```python
from build123d import *

# Parameters (mm, degrees)
CROQUIS1_W              = 68
CROQUIS1_H              = 64
CROQUIS1_W_2            = 61.625
CROQUIS1_H_2            = 58
SALIENTE_EXTRUIR1_DEPTH = 25
SALIENTE_EXTRUIR2_DEPTH = 160
SALIENTE_EXTRUIR3_DEPTH = 61
SALIENTE_EXTRUIR5_DEPTH = 3
CROQUIS4_W              = 100
CROQUIS4_H              = 30
CORTAR_EXTRUIR1_DEPTH   = 83
CHAFL_N1_SIZE           = 2
CHAFL_N1_SIZE2          = 57.272506566
CROQUIS1_2_W            = 68
CROQUIS1_2_H            = 64
CROQUIS1_2_W_2          = 61.625
CROQUIS1_2_H_2          = 58
SALIENTE_EXTRUIR6_DEPTH = 5
CROQUIS5_W              = 40
CROQUIS5_H              = 60
CORTAR_EXTRUIR2_DEPTH   = 90
CROQUIS1_4_W            = 68
CROQUIS1_4_H            = 10
CROQUIS1_4_R            = 2
SALIENTE_EXTRUIR7_DEPTH = 5
CROQUIS6_W              = 75.447981844
CROQUIS6_H              = 15
CORTAR_EXTRUIR3_DEPTH   = 5
CHAFL_N2_SIZE           = 30
CHAFL_N2_SIZE_2         = 1.572233378
CHAFL_N3_SIZE           = 5
CHAFL_N3_SIZE2          = 0.881634904
CROQUIS7_W              = 58
CROQUIS7_H              = 20
CORTAR_EXTRUIR4_DEPTH   = 40
CROQUIS8_W              = 58
CROQUIS8_H              = 40
CORTAR_EXTRUIR5_DEPTH   = 10
REDONDEO2_R             = 5
CORTAR_EXTRUIR6_DEPTH   = 70
REDONDEO5_R             = 5


with BuildPart() as part:
    # Croquis1 → Saliente-Extruir1 (new body)
    with BuildSketch(Plane(origin=(0, 0, 0), x_dir=(1, 0, 0), z_dir=(0, 1, 0))):
        Rectangle(CROQUIS1_W, CROQUIS1_H)
        Rectangle(CROQUIS1_W_2, CROQUIS1_H_2, mode=Mode.SUBTRACT)
    extrude(amount=SALIENTE_EXTRUIR1_DEPTH)

    # Croquis2 → Saliente-Extruir2 (add)
    with BuildSketch(Plane(origin=(0, 25, 0), x_dir=(1, 0, 0), z_dir=(0, 1, 0))):
        Polygon((0, 29), (0, 32), (34, 32), (34, -32), (0, -32), (0, -29), (30.8125, -29), (30.8125, 29), align=None)
    extrude(amount=SALIENTE_EXTRUIR2_DEPTH)



with BuildPart() as body_2:
    # Croquis3 → Saliente-Extruir3 (new body)
    with BuildSketch(Plane(origin=(0, 0, 29), x_dir=(-1, 0, 0), z_dir=(0, 0, -1))):
        Polygon((0, 155), (5, 155), (2, 85), (0, 85), align=None)
    extrude(amount=SALIENTE_EXTRUIR3_DEPTH)


with BuildPart() as part_1:
    add(part.part)

    add(body_2.part)  # Saliente-Extruir5 merges body 2
    # Croquis3<4> → Saliente-Extruir5 (add)
    with BuildSketch(Plane(origin=(0, 0, 29), x_dir=(-1, 0, 0), z_dir=(0, 0, -1))):
        Polygon((0, 155), (5, 155), (2, 85), (0, 85), align=None)
    extrude(amount=-SALIENTE_EXTRUIR5_DEPTH)

    # Croquis4 → Cortar-Extruir1 (cut)
    with BuildSketch(Plane(origin=(0, 0, -32), x_dir=(-1, 0, 0), z_dir=(0, 0, -1))):
        with Locations((19, 170)):
            Rectangle(CROQUIS4_W, CROQUIS4_H)
    extrude(amount=-CORTAR_EXTRUIR1_DEPTH, mode=Mode.SUBTRACT)

    # Chaflán1
    chafl_n1_edges = [part_1.edges().sort_by_distance(p)[0] for p in [
        (0, 155, 0),
    ]]
    chafl_n1_side = [part_1.faces().sort_by_distance(p)[0] for p in [
        (13, 155, -31.26569761),
    ]]
    chamfer(chafl_n1_edges, length=CHAFL_N1_SIZE, length2=CHAFL_N1_SIZE2, reference=chafl_n1_side[0])

    # Croquis1<2> → Saliente-Extruir6 (add)
    # profile 1 of 2: a face of its own
    with BuildSketch(Plane(origin=(0, 0, 0), x_dir=(1, 0, 0), z_dir=(0, 1, 0))):
        Rectangle(CROQUIS1_2_W, CROQUIS1_2_H)
        Rectangle(CROQUIS1_2_W_2, CROQUIS1_2_H_2, mode=Mode.SUBTRACT)
    # profile 2 of 2: a face of its own
    with BuildSketch(Plane(origin=(0, 0, 0), x_dir=(1, 0, 0), z_dir=(0, 1, 0))):
        Rectangle(CROQUIS1_2_W_2, CROQUIS1_2_H_2)
    extrude(amount=SALIENTE_EXTRUIR6_DEPTH)

    # Croquis5 → Cortar-Extruir2 (cut)
    with BuildSketch(Plane(origin=(0, 0, -32), x_dir=(-1, 0, 0), z_dir=(0, 0, -1))):
        with Locations((-11, 55)):
            Rectangle(CROQUIS5_W, CROQUIS5_H)
    extrude(amount=-CORTAR_EXTRUIR2_DEPTH, mode=Mode.SUBTRACT)

    # Croquis1<4> → Saliente-Extruir7 (add)
    # profile 1 of 2: a face of its own
    with BuildSketch(Plane(origin=(0, 0, 0), x_dir=(1, 0, 0), z_dir=(0, 1, 0))):
        with Locations((0, 37)):
            Rectangle(CROQUIS1_4_W, CROQUIS1_4_H)
        with Locations(Location((0, 37, 0), (0, 0, 270))):
            Circle(CROQUIS1_4_R, mode=Mode.SUBTRACT)
    # profile 2 of 2: a face of its own
    with BuildSketch(Plane(origin=(0, 0, 0), x_dir=(1, 0, 0), z_dir=(0, 1, 0))):
        with Locations((0, -37)):
            Rectangle(CROQUIS1_4_W, CROQUIS1_4_H)
        with Locations(Location((0, -37, 0), (0, 0, 270))):
            Circle(CROQUIS1_4_R, mode=Mode.SUBTRACT)
    extrude(amount=SALIENTE_EXTRUIR7_DEPTH)

    # Croquis6 → Cortar-Extruir3 (cut)
    with BuildSketch(Plane.ZY.offset(-31)):
        with Locations((5.723990922, 177.5)):
            Rectangle(CROQUIS6_W, CROQUIS6_H)
    extrude(amount=-CORTAR_EXTRUIR3_DEPTH, mode=Mode.SUBTRACT)

    # Chaflán2
    # the kernel refuses this chamfer: 30, 1.572233378 mm, written as the material it takes off along each edge
    with BuildSketch(Plane(origin=(31, 170, -109.996046635), x_dir=(-0.002013023422382327, -0.9999979738662979, 0), z_dir=(0, 0, 1))) as chafl_n2_piece_1_section:
        Polygon((CHAFL_N2_SIZE * 0.999997973866, CHAFL_N2_SIZE * 0.00201302342238), (-CHAFL_N2_SIZE_2 * 0.00201302342301, CHAFL_N2_SIZE_2 * 0.999997974179), (0, 0), align=None)
    chafl_n2_piece_1 = extrude(amount=219.992093269, mode=Mode.PRIVATE)
    chafl_n2_piece_1 = split(chafl_n2_piece_1, bisect_by=Plane(origin=(31.611424092, 155, 0), z_dir=(0, 1, 0)), keep=Keep.TOP, mode=Mode.PRIVATE)
    add(chafl_n2_piece_1, mode=Mode.SUBTRACT)

    # Chaflán3
    chafl_n3_edges = [part_1.edges().sort_by_distance(p)[0] for p in [
        (30.8125, 155, 0),
    ]]
    chafl_n3_side = [part_1.faces().sort_by_distance(p)[0] for p in [
        (30.8125, 120, 0),
    ]]
    chamfer(chafl_n3_edges, length=CHAFL_N3_SIZE, length2=CHAFL_N3_SIZE2, reference=chafl_n3_side[0])

    # Croquis7 → Cortar-Extruir4 (cut)
    with BuildSketch(Plane.ZY.offset(34)):
        with Locations((0, 15)):
            Rectangle(CROQUIS7_W, CROQUIS7_H)
    extrude(amount=-CORTAR_EXTRUIR4_DEPTH, mode=Mode.SUBTRACT)

    # Croquis8 → Cortar-Extruir5 (cut)
    with BuildSketch(Plane(origin=(1.639845182, 0.070279079, 0), x_dir=(0, 0, 1), z_dir=(-0.9990828958176697, -0.04281783839218585, 0))):
        with Locations((0, 135.071938044)):
            Rectangle(CROQUIS8_W, CROQUIS8_H)
    extrude(amount=-CORTAR_EXTRUIR5_DEPTH, mode=Mode.SUBTRACT)

    # Redondeo2
    # the kernel refuses this fillet: 5 mm, written as the material it takes off along each edge
    with BuildSketch(Plane(origin=(-0.608459404, 115.151491041, 29), x_dir=(0.034899496702498145, -0.9993908270190959, 0), z_dir=(0, 0, -1))) as redondeo2_piece_1:
        with BuildLine():
            CenterArc((4.451052559, 5), REDONDEO2_R, 207.629976372, 62.370023628)
            Line((0.021247221, 2.681201893), (0, 0))
            Line((0, 0), (4.451052559, 0))
        make_face()
    extrude(amount=58, mode=Mode.SUBTRACT)

    # Croquis9 → Cortar-Extruir6 (cut)
    with BuildSketch(Plane.XY.offset(32)):
        Polygon((-5, 155), (-4.15481256, 135.278959735), (31.786116689, 135.278959735), (31.786116689, 137.80344281), (31.786116689, 155), (-4.263004692, 155), align=None)
    extrude(amount=-CORTAR_EXTRUIR6_DEPTH, mode=Mode.SUBTRACT)

    # Redondeo5
    # the kernel refuses this fillet: 5 mm, written as the material it takes off along each edge
    with BuildSketch(Plane(origin=(30.8125, 135.278959735, 29), x_dir=(0, 0, 1), z_dir=(-1, 0, 0))) as redondeo5_piece_1_section:
        with BuildLine():
            CenterArc((5, -4.582575695), REDONDEO5_R, 113.578178478, 66.421821522)
            Line((0, -4.582575695), (-0.1, -4.582575695))
            Line((-0.1, -4.582575695), (-0.1, 0))
            Line((-0.1, 0), (0, 0.1))
            ThreePointArc((0, 0.1), (1.5, 0.1), (2.96, 0.091651514))
            Line((2.96, 0.091651514), (3, 0))
        make_face()
    redondeo5_piece_1 = extrude(amount=46.423751797, mode=Mode.PRIVATE)
    redondeo5_piece_1 = split(redondeo5_piece_1, bisect_by=Plane(origin=(-4.075030571, 133.417379989, 29.7763393), z_dir=(0.9990828958176697, 0.042817838392185836, 0)), keep=Keep.TOP, mode=Mode.PRIVATE)
    add(redondeo5_piece_1, mode=Mode.SUBTRACT)
    with BuildSketch(Plane(origin=(-15.611251797, 135.278959735, -29), x_dir=(0, -1, 0), z_dir=(1, 0, 0))) as redondeo5_piece_2_section:
        with BuildLine():
            CenterArc((4.582575695, 5), REDONDEO5_R, 203.578178478, 66.421821522)
            Line((0, 3), (-0.091651514, 2.96))
            ThreePointArc((-0.091651514, 2.96), (-0.1, 1.5), (-0.1, 0))
            Line((-0.1, 0), (0, -0.1))
            Line((0, -0.1), (4.582575695, -0.1))
            Line((4.582575695, -0.1), (4.582575695, 0))
        make_face()
    redondeo5_piece_2 = extrude(amount=46.423751797, mode=Mode.PRIVATE)
    redondeo5_piece_2 = split(redondeo5_piece_2, bisect_by=Plane(origin=(-4.075030571, 133.417379989, -29.7763393), z_dir=(0.9990828958176697, 0.042817838392185836, 0)), keep=Keep.TOP, mode=Mode.PRIVATE)
    add(redondeo5_piece_2, mode=Mode.SUBTRACT)
    with BuildSketch(Plane(origin=(30.8125, 135.278959735, -29), x_dir=(1, 0, 0), z_dir=(0, 0, 1))) as redondeo5_piece_3:
        with BuildLine():
            CenterArc((5, -2.964496152), REDONDEO5_R, 143.636982553, 36.363017447)
            Line((0, -2.964496152), (-0.1, -2.964496152))
            Line((-0.1, -2.964496152), (-0.1, 0))
            Line((-0.1, 0), (0, 0.1))
            ThreePointArc((0, 0.1), (0.486808345, 0.1), (0.893089023, 0.059289923))
            Line((0.893089023, 0.059289923), (0.973616689, 0))
        make_face()
    extrude(amount=58, mode=Mode.SUBTRACT)
    with BuildSketch(Plane(origin=(30.8125, 135.278959735, -29), x_dir=(1, 0, 0), z_dir=(0, 0, 1))) as redondeo5_piece_4a_section:
        with BuildLine():
            CenterArc((5, -2.964496152), REDONDEO5_R, 143.636982553, 36.363017447)
            Line((0, -2.964496152), (-0.1, -2.964496152))
            Line((-0.1, -2.964496152), (-0.1, 0))
            Line((-0.1, 0), (0, 0.1))
            ThreePointArc((0, 0.1), (0.486808345, 0.1), (0.893089023, 0.059289923))
            Line((0.893089023, 0.059289923), (0.973616689, 0))
        make_face()
    redondeo5_piece_4a = extrude(amount=65.41124038, mode=Mode.PRIVATE)
    redondeo5_piece_4a = split(redondeo5_piece_4a, bisect_by=Plane(origin=(31.030991271, 134.436005592, 29), z_dir=(0, 0, 1)), keep=Keep.TOP, mode=Mode.PRIVATE)
    with BuildSketch(Plane(origin=(42.268939237, 135.278959735, 29), x_dir=(0, 0, 1), z_dir=(-1, 0, 0))) as redondeo5_piece_4b_section:
        with BuildLine():
            CenterArc((5, -4.582575695), REDONDEO5_R, 113.578178478, 66.421821522)
            Line((0, -4.582575695), (-0.1, -4.582575695))
            Line((-0.1, -4.582575695), (-0.1, 0))
            Line((-0.1, 0), (0, 0.1))
            ThreePointArc((0, 0.1), (1.5, 0.1), (2.96, 0.091651514))
            Line((2.96, 0.091651514), (3, 0))
        make_face()
    redondeo5_piece_4b = extrude(amount=57.880191035, mode=Mode.PRIVATE)
    redondeo5_piece_4b = split(redondeo5_piece_4b, bisect_by=Plane(origin=(30.8125, 134.163022014, 29.775816439), z_dir=(1, 0, 0)), keep=Keep.TOP, mode=Mode.PRIVATE)
    redondeo5_piece_4 = redondeo5_piece_4a & redondeo5_piece_4b
    add(redondeo5_piece_4, mode=Mode.SUBTRACT)
    with BuildSketch(Plane(origin=(-15.611251797, 135.278959735, -29), x_dir=(0, -1, 0), z_dir=(1, 0, 0))) as redondeo5_piece_5a_section:
        with BuildLine():
            CenterArc((4.582575695, 5), REDONDEO5_R, 203.578178478, 66.421821522)
            Line((0, 3), (-0.091651514, 2.96))
            ThreePointArc((-0.091651514, 2.96), (-0.1, 1.5), (-0.1, 0))
            Line((-0.1, 0), (0, -0.1))
            Line((0, -0.1), (4.582575695, -0.1))
            Line((4.582575695, -0.1), (4.582575695, 0))
        make_face()
    redondeo5_piece_5a = extrude(amount=57.880191035, mode=Mode.PRIVATE)
    redondeo5_piece_5a = split(redondeo5_piece_5a, bisect_by=Plane(origin=(30.8125, 134.163022014, -29.775816439), z_dir=(1, 0, 0)), keep=Keep.TOP, mode=Mode.PRIVATE)
    with BuildSketch(Plane(origin=(30.8125, 135.278959735, -36.41124038), x_dir=(1, 0, 0), z_dir=(0, 0, 1))) as redondeo5_piece_5b_section:
        with BuildLine():
            CenterArc((5, -2.964496152), REDONDEO5_R, 143.636982553, 36.363017447)
            Line((0, -2.964496152), (-0.1, -2.964496152))
            Line((-0.1, -2.964496152), (-0.1, 0))
            Line((-0.1, 0), (0, 0.1))
            ThreePointArc((0, 0.1), (0.486808345, 0.1), (0.893089023, 0.059289923))
            Line((0.893089023, 0.059289923), (0.973616689, 0))
        make_face()
    redondeo5_piece_5b = extrude(amount=65.41124038, mode=Mode.PRIVATE)
    redondeo5_piece_5b = split(redondeo5_piece_5b, bisect_by=Plane(origin=(31.030991271, 134.436005592, -29), z_dir=(0, 0, -1)), keep=Keep.TOP, mode=Mode.PRIVATE)
    redondeo5_piece_5 = redondeo5_piece_5a & redondeo5_piece_5b
    add(redondeo5_piece_5, mode=Mode.SUBTRACT)


solid = part_1.part
```
Design review of the part built by this model. Coordinates are the model's own, in mm. A direction names the side the tool comes from. Coordinates: 2 decimals unless noted, no trailing zeros. Write each loop counter-clockwise with the first axis right and the second up, starting at its lowest first coordinate (ties: lowest second). Pieces come first, ordered by that corner, then holes.
1) Mouldability with a two-part tool opening along Y and no side actions: class faces 4 (the cylindrical face through (0, 2, 35)), 5 (the flat face through (-2, 25, -31)), 6 (the flat face through (32.174, 162.395, -0.448)) as +Y half, -Y half, draft (parallel to the pull), parting line (faces both ways), or undercut.
2) To check wall thickness, follow L1, parallel to X at y = 3.85, z = 37; L2, parallel to Y at x = -29.5, z = -13; L3, parallel to X at y = 126.5, z = 0.5. State the ranges of each line that lie inside material, in increasing order.
3) Add section A-A (x = 21). Write out the cut boundary in (y, z), plus the area to 3 significant figures.
4) Add section C-C (x = -26). Write out the cut boundary in (y, z).
5) Add section D-D (z = 20). Write out the cut boundary in (x, y).
6) Add section B-B (z = -37). Write out the cut boundary in (x, y), plus the area to 3 significant figures.
7) Insertion check: pin 1 (6 mm diameter, centred on x = -9, z = -32, fed in from -Y); pin 2 (10 mm diameter, centred on x = 3.5, y = 11.5, fed in from +Z); pin 3 (2.5 mm diameter, centred on x = 0, z = -37, fed in from -Y); pin 4 (4 mm diameter, centred on y = 112.5, z = -23, fed in from -X). Each pin has a flat end and moves straight along its axis. Give the tip position at first contact, or say it passes through.
8) Machinability: for faces 1 (the flat face through (30.812, 108, 0)), 2 (the flat face through (31.786, 145, 0)), 3 (the cylindrical face through (13.56, 133.47, -29.84)), which of the approach directions +Z, -Z, +X, -X, +Y, -Y give a long, thin tool a straight path to every point of the face, cutting with its end or side? Answer none if there is none.
Check result:
1. face 4: draft
1. face 5: undercut
1. face 6: +Y half
2. L1: x = -34 to -2, 2 to 34
2. L2: y = 0 to 5
2. L3: x = 30.81 to 34
3. outline: (0, -42) - (5, -42) - (5, -32) - (25, -32) - (25, -29) - (5, -29) - (5, 29) - (25, 29) - (25, 32) - (5, 32) - (5, 42) - (0, 42) - close; (85, -32) - (135.28, -32) arc R5 ccw to (130.7, -29) - (85, -29) - close; (85, 29) - (130.7, 29) arc R5 ccw to (135.28, 32) - (85, 32) - close
3. area: 834 mm2
4. outline: (0, -42) - (5, -42) - (5, -32) - (25, -32) - (25, -29) - (5, -29) - (5, 29) - (25, 29) - (25, 32) - (5, 32) - (5, 42) - (0, 42) - close
5. outline: (-34, 0) - (34, 0) - (34, 170) - (32.57, 170) - (31.79, 155) - (31.79, 135.28) arc R5 ccw to (30.81, 132.31) - (30.81, 85) - (31, 85) - (31, 25) - (30.81, 25) - (30.81, 5) - (-34, 5) - close; (-3.29, 115.04) - (-2, 85) - (0, 85) - (0, 97.73) - (-0.45, 110.7) arc R5 ccw to start
6. outline: (-34, 0) - (-2, 0) - (-2, 5) - (-34, 5) - close; (2, 0) - (34, 0) - (34, 5) - (2, 5) - close
6. area: 320 mm2
7. pin 1: stops at y = 0
7. pin 2: stops at z = 32
7. pin 3: passes through
7. pin 4: stops at x = -3.26
8. face 1: +Y
8. face 2: +Z, -Z, -X, +Y
8. face 3: -X, +Y
